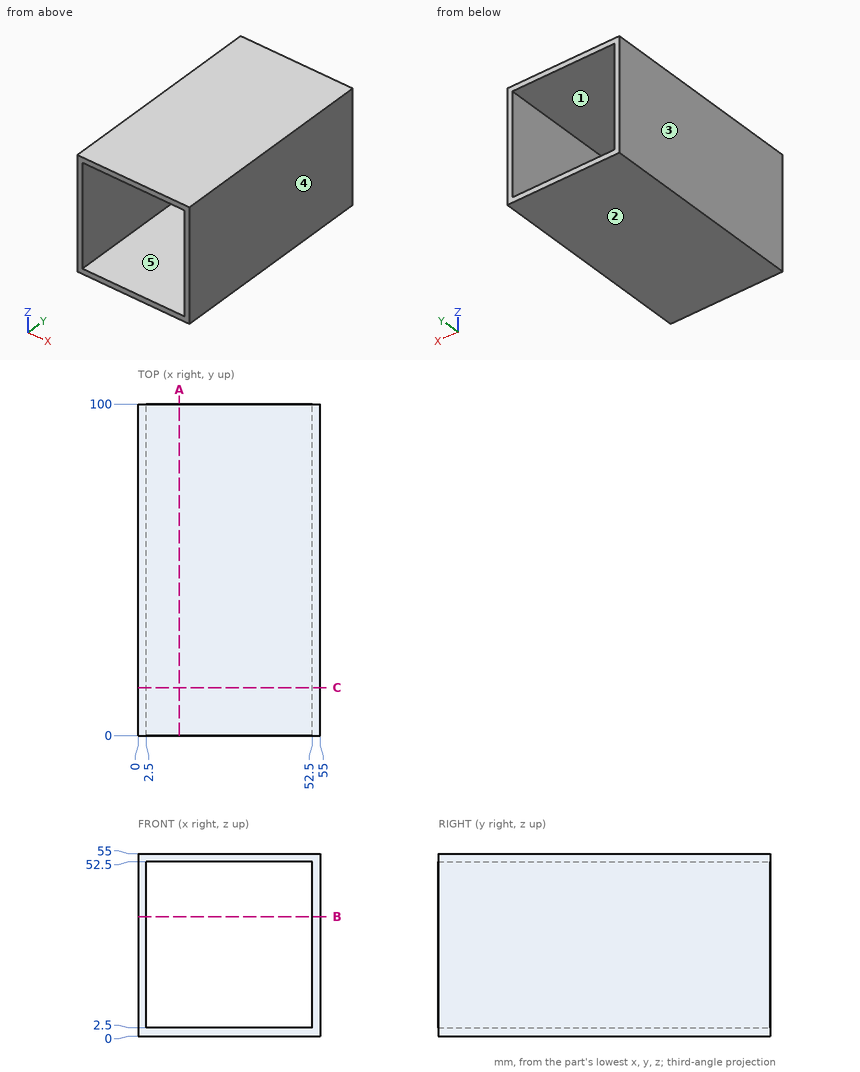
Drawing for the job (mm, zero at the part's lowest x, y, z). A direction names the side the tool comes from. Round coordinates to 2 decimals unless told otherwise and drop trailing zeros. Order: outer loops, then holes, each group sorted by start corner. A loop starts at its lowest first (then second) coordinate and runs counter-clockwise, first axis right, second up.
Item 1: Saw through at C-C on y = 14.5. Write the cut outline in (x, z).
Item 2: Pin check, flat tip, straight feed: pin 1 (12 mm diameter, centred on x = 44, z = 34.5, fed in from +Y). Stop position of the tip, or through.
Item 3: Mould opens along X. For the marked faces 3, 4 and 5 say: pulls with the +X half, pulls with the -X half, needs draft (parallel to the pull), parting line crosses it, or undercut.
Item 4: Probe line 1 along Z through (x, y) = (18, 87.5). List the from-to ranges inside material, lowest first.
Item 5: Tool access for the marked faces 1 and 2: list every direction of +Z, -Z, +X, -X, +Y, -Y with a clear straight run to the whole face (end or side of a thin tool).
Item 6: Saw through at B-B on z = 36. Write the cut outline in (x, y), then the cut area to 3 significant figures.
Item 7: Saw through at A-A on x = 12.5. Write the cut outline in (y, z), then the cut area to 3 significant figures.
Reported:
1. outline: (0, 0) - (55, 0) - (55, 55) - (0, 55) - close; hole (2.5, 2.5) - (52.5, 2.5) - (52.5, 52.5) - (2.5, 52.5) - close
2. pin 1: passes through
3. face 3: pulls with the -X half
3. face 4: pulls with the +X half
3. face 5: undercut
4. line 1: z = 0 to 2.5, 52.5 to 55
5. face 1: +Y, -Y
5. face 2: -Z, +X, -X, +Y, -Y
6. outline: (0, 0) - (2.5, 0) - (2.5, 100) - (0, 100) - close; (52.5, 0) - (55, 0) - (55, 100) - (52.5, 100) - close
6. area: 500 mm2
7. outline: (0, 0) - (100, 0) - (100, 2.5) - (0, 2.5) - close; (0, 52.5) - (100, 52.5) - (100, 55) - (0, 55) - close
7. area: 500 mm2
